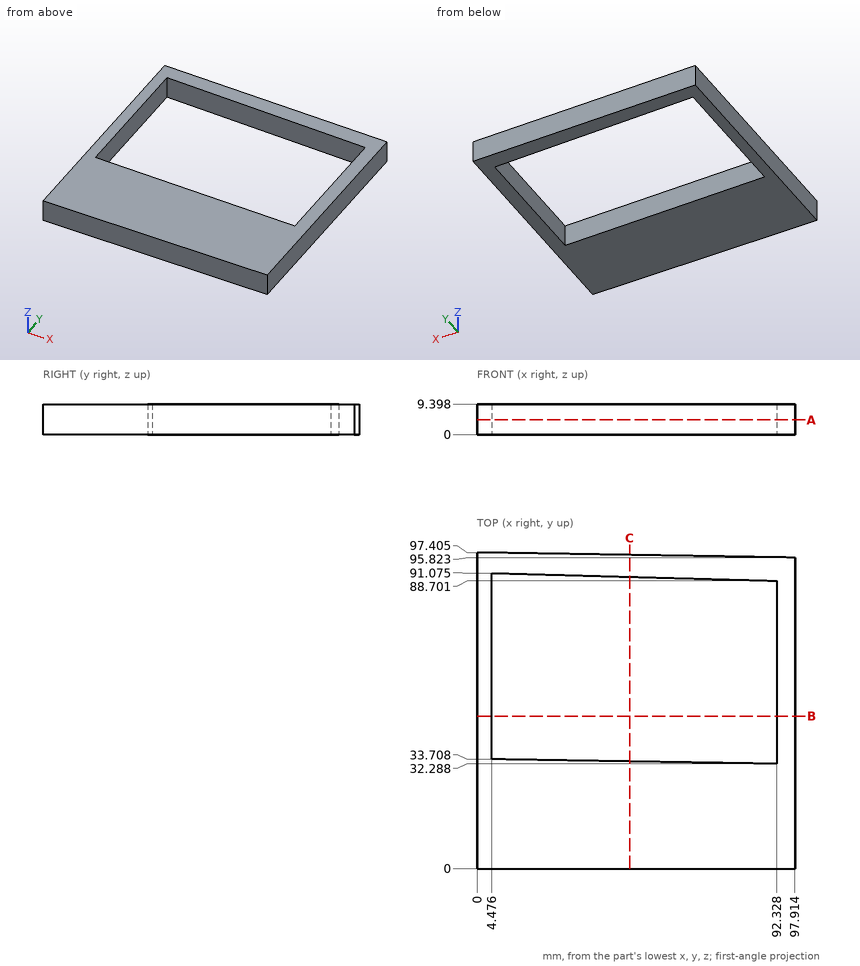
Print and shaded views of the part. All mm, measured from the part's lowest x, y and z. Coordinates: 2 decimals unless noted, no trailing zeros. Write each loop counter-clockwise with the first axis right and the second up, starting at its lowest first coordinate (ties: lowest second). Pieces come first, ordered by that corner, then holes. Notation, with made-up numbers: (24, 47) - (83, 47) arc R25 cw to (83, 69) - close; hole circle Ø11 at (69, 16). An arc over 180 degrees is marked (long way). One line per question, with ' | ' between items. Start each with the question number.
Q1. Cut at B-B, the plane y = 47. List the corners of the cut face in (x, z) (1 decimal).
Q2. Cut at C-C, the plane x = 47. List the corners of the cut face in (y, z) (1 decimal).
Q3. Cut at A-A, the plane z = 4.5. List the corners of the cut face in (x, y) (1 decimal), then the cut area to 3 significant figures.
Q4. Pin check, flat tips, straight feed: pin 1 (5 mm diameter, centred on x = 17, z = 8, fed in from +Y); pin 2 (2 mm diameter, centred on x = 80, z = 7.5, fed in from +Y). Stop position of each tip, or through.
Q5. Drill centre lines: line 1 (X direction, y = 67, z = 3) (1 decimal); line 2 (Y direction, x = 52, z = 8.25) (1 decimal); line 3 (Y direction, x = 42, z = 6.5). Where is each one in solid material? Low to high. Write a range as [from, to].
Answer below:
1) outline: (0, 0) - (4.5, 0) - (4.5, 9.4) - (0, 9.4) - close; (92.3, 0) - (97.9, 0) - (97.9, 9.4) - (92.3, 9.4) - close
2) outline: (0, 0) - (33, 0) - (33, 9.4) - (0, 9.4) - close; (89.9, 0) - (96.6, 0) - (96.6, 9.4) - (89.9, 9.4) - close
3) outline: (0, 0) - (97.9, 0) - (97.9, 95.8) - (0, 97.4) - close; hole (4.5, 33.7) - (92.3, 32.3) - (92.3, 88.7) - (4.5, 91.1) - close | area: 4,460 mm^2
4) pin 1: y = 97.17 | pin 2: y = 96.13
5) line 1: [0, 4.5], [92.3, 97.9] | line 2: [0, 32.9], [89.8, 96.6] | line 3: [0, 33.1], [90.06, 96.73]
